Geometry: final body of the model. Coordinates: model frame, mm. Round coordinates to 2 decimals unless told otherwise and drop trailing zeros. Order: outer loops, then holes, each group sorted by start corner. A loop starts at its lowest first (then second) coordinate and runs counter-clockwise, first axis right, second up. Notation, with made-up numbers: M 29,-28 L 62,-28 A18 cw 62,-9 Z; hole C 74,-39.75 d1. An arc over 180 degrees is marked long. Put each result on its own line as item: value. Start each with the question number.
1) First-contact query: P1, Ø12.5, axis at x = -10, y = 0, coming from the -Z side; P2, Ø1, axis at y = 13, z = 0.5, coming from the +X side. Flat tips, straight axial feed; report the tip coordinate or a pass-through.
2) Section D-D, the plane x = -26. Return loops of the section in (y, z).
3) Section A-A, the plane y = 15. Return loops of the section in (x, z).
4) Material intervals for probe 1 along X at (y, z) = (-16, 0.6); probe 2 along Y at (x, z) = (24.6, 1.4); probe 3 along X at (y, z) = (16, 1.45), sorted ascending. Write a range as [from, to].
5) Section B-B, the plane x = -13. Return loops of the section in (y, z).
6) Section C-C, the plane z = 0.7. Count the separate pieces of the cut face and the enclosed holes in it, then the cut area to 3 significant figures.
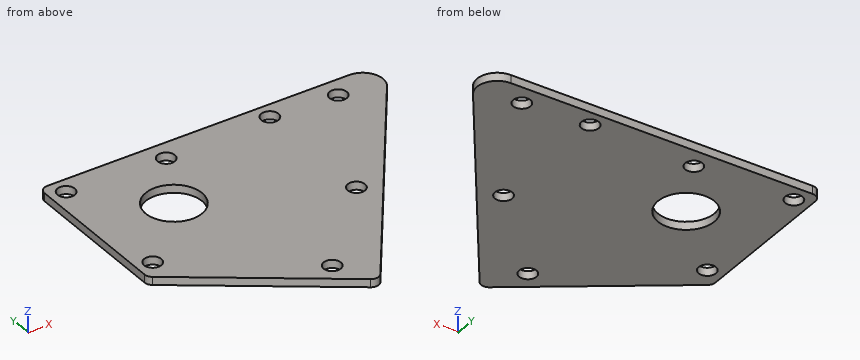
Autodesk Inventor part; units mm, degrees
ref_plane "YZ Plane" through (0, 0, 0) normal (1, 0, 0) x (0, 1, 0)
ref_plane "XZ Plane" through (0, 0, 0) normal (0, 1, 0) x (-1, 0, 0)
ref_plane "XY Plane" through (0, 0, 0) normal (0, 0, 1) x (1, 0, 0)
sketch "スケッチ1" plane through (0, 0, 0) normal (0, 0, 1) x (1, 0, 0)
  line L0 (-30, -20) -> (28.6, -20)
  line L1 (28.6, -20) -> (28.6, 20)
  line L2 (28.6, 20) -> (-30, 20)
  line L3 (-30, 20) -> (-30, -20)
  point P0 (0, 0)
  dimension "d1" = 40
  dimension "d28" = 30
  dimension "d29" = 28.6
  dimension "d32" = 20
extrude "プレート1" add sketch "スケッチ1" along normal blind 2
sketch "スケッチ2" plane through (0, 0, 2) normal (0, 0, 1) x (1, 0, 0)
  line L0 (-24, -5) -> (24.6, -5)
  line L1 (24.6, -5) -> (24.6, 5)
  line L2 (24.6, 5) -> (-24, 5)
  line L3 (-24, 5) -> (-24, -5)
  line L4 (-24, -5) -> (24.6, 5) construction
  line L5 (24.6, -5) -> (-24, 5) construction
  line L6 (28.6, -20) -> (-30, -20)
  line L7 (-30, -20) -> (-30, 20)
  line L8 (28.6, -20) -> (-30, -20)
  line L9 (28.6, 20) -> (28.6, -20)
  line L10 (-30, 20) -> (28.6, 20)
  circle A0 centre (-10, 0) radius 7
  point P0 (0.3, 0)
  point P1 (0.3, 0)
  point P2 (0.3, 0)
  point P3 (0, 0)
  dimension "GapSize" = 2
  dimension "d3" = 48.6
  dimension "d5" = 10
  dimension "d8" = 20
  dimension "d16" = 14
  dimension "d30" = 20
  dimension "d31" = 14
extrude "押し出し1" cut sketch "スケッチ2" against normal blind 10 contours A0 L2 L0 | L0 A0 | A0 L2
sketch "スケッチ3" plane through (0, 0, 2) normal (0, 0, 1) x (1, 0, 0)
  line L0 (-30, 20) -> (28.6, 20)
  line L1 (-30, -20) -> (-30, 20)
  line L2 (28.6, -20) -> (-30, -20)
  line L3 (28.6, 20) -> (28.6, -20)
  line L4 (24.6, 16) -> (-26, 16)
  line L5 (-26, 16) -> (-26, -16)
  line L6 (-26, -16) -> (24.6, -16)
  line L7 (24.6, -16) -> (24.6, 16)
  point P0 (0, 0)
  dimension "d19" = 4
hole "穴2" at (-26, 16, 2) at (-26, -16, 2) at (24.6, 16, 2) at (24.6, -16, 2) direction (0, 0, -1) diameter 4.3 end through all
sketch "スケッチ4" plane through (0, 0, 2) normal (0, 0, 1) x (1, 0, 0)
  line L0 (-30, -20) -> (28.6, -20)
  line L1 (28.6, -20) -> (56.6083, 20)
  line L2 (28.6, 20) -> (28.6, -20)
  line L3 (28.6, 20) -> (56.6083, 20)
  line L4 (-30, -20) -> (9.3212, -47.533)
  line L5 (28.6, -20) -> (9.3212, -47.533)
  point P0 (0, 0)
  dimension "d33" = 35
  dimension "d34" = 35
sheet face with bend "面2" sketch "スケッチ4" thickness 2 toward (0, 0, -1) bend radius 2
bend "曲げ1"
sketch "スケッチ5" plane through (0, 0, 2) normal (0, 0, 1) x (1, 0, 0)
  line L0 (-30, -20) -> (9.3212, -47.533)
  line L1 (9.3212, -47.533) -> (56.6083, 20)
  line L2 (56.6083, 20) -> (-30, 20)
  point P0 (0, 0)
  point P1 (3.9976, -37.7015)
  point P2 (40.8995, 15)
  point P3 (-1.8276, 15)
  dimension "d40" = 5
  dimension "d41" = 10
  dimension "d42" = 10
  dimension "d43" = 5
  dimension "d44" = 5
  dimension "d45" = 45
hole "穴3" at (3.9976, -37.7015, 2) at (40.8995, 15, 2) at (-1.8276, 15, 2) direction (0, 0, -1) diameter 4.3 end through all
fillet "フィレット1" radius 2 3 edges at (-30, 20, 1) (-30, -20, 1) (9.3212, -47.533, 1)
fillet "フィレット2" radius 5 1 edges at (56.6083, 20, 1)
equation "\"GapSize\" = Thickness"
equation "\"d51\" = Thickness"
equation "\"d2\" = Thickness"
equation "\"d35\" = BendRadius"
equation "\"d36\" = BendReliefWidth"
equation "\"d38\" = MinimumRemnant"
equation "\"d37\" = BendReliefDepth"
equation "\"d39\" = TransitionRadius"
equation "\"BendRadius\" = Thickness"
equation "\"BendReliefWidth\" = Thickness"
equation "\"BendReliefDepth\" = 0.5 * Thickness"
equation "\"CornerReliefSize\" = 4 * Thickness"
equation "\"MinimumRemnant\" = 2 * Thickness"
equation "\"TransitionRadius\" = BendRadius"
equation "\"JacobiRadiusSize\" = BendRadius"
properties part number "s_carbon_plate4" material "CFRP"
Result sheet:
1. P1: passes through
1. P2: stops at x = 51.77
2. outline: M -22.8,0 L -18.15,0 L -18.15,2 L -22.8,2 Z; M -13.85,0 L 13.85,0 L 13.85,2 L -13.85,2 Z; M 18.15,0 L 20,0 L 20,2 L 18.15,2 Z
3. outline: M -30,0 L -27.9,0 L -27.9,2 L -30,2 Z; M -24.1,0 L -3.98,0 L -3.98,2 L -24.1,2 Z; M 0.32,0 L 22.7,0 L 22.7,2 L 0.32,2 Z; M 26.5,0 L 38.75,0 L 38.75,2 L 26.5,2 Z; M 43.05,0 L 52,0 L 52,2 L 43.05,2 Z
4. probe 1: x = [-30, -28.15], [-23.85, 22.45], [26.75, 31.4]
4. probe 2: y = [-25.71, -18.15], [-13.85, 13.85], [18.15, 20]
4. probe 3: x = [-30, -28.15], [-23.85, -3.73], [0.08, 22.45], [26.75, 39], [42.8, 51.9]
5. outline: M -31.9,0 L -6.32,0 L -6.32,2 L -31.9,2 Z; M 6.32,0 L 20,0 L 20,2 L 6.32,2 Z
6. separate pieces: 1
6. enclosed holes: 8
6. area: 3,430 mm2
